The drawing under review shows one solid part. Ordinate dimensions are in mm from its lowest x, y, z. Give positions to 0.01 mm unless a question says otherwise; leave off trailing zeros. Order: outer loops, then holes, each group sorted by start corner. A loop starts at its lowest first (then second) coordinate and runs counter-clockwise, first axis right, second up. Notation, with made-up numbers: (64, -22.75) - (88, -22.75) arc R38 cw to (88, 15.25) - close; hole circle Ø10 at (-31, 58). An arc over 180 degrees is marked (long way). Write item = value, one per line. Start each with the question number.
1. We need section C-C, the plane z = 8.75. Give the boundary of the cut face in (x, y), and give its area (3 significant figures).
2. For P1, Ø0.9, axis at x = 2.5, y = 3, coming from the +Z side; P2, Ø2, axis at y = 1, z = 12, coming from the -X side; P3, Ø0.8, axis at y = 2, z = 0.5, coming from the -X side, all flat-tipped, find the tip position at first contact; note any pin that passes through.
3. Mouldability with a two-part tool opening along Y and no side actions: class the marked faces 1, 2 and 3 as pulls with the +Y half, pulls with the -Y half, needs draft (parallel to the pull), parting line crosses it, or undercut.
4. Wall thickness on probe 1 along Y at (x, z) = (3, 10); probe 2 along Z at (x, y) = (2.9, 1.65); probe 3 along Y at (x, z) = (4.1, 10.5): over which ranges is each line inside the solid? List them lowest first.
5. We need section D-D, the plane z = 4.25. Give the boundary of the cut face in (x, y).
6. We need section B-B, the plane x = 3. Give the boundary of the cut face in (y, z), and give its area (4 significant figures).
7. We need section A-A, the plane y = 3. Give the boundary of the cut face in (x, z).
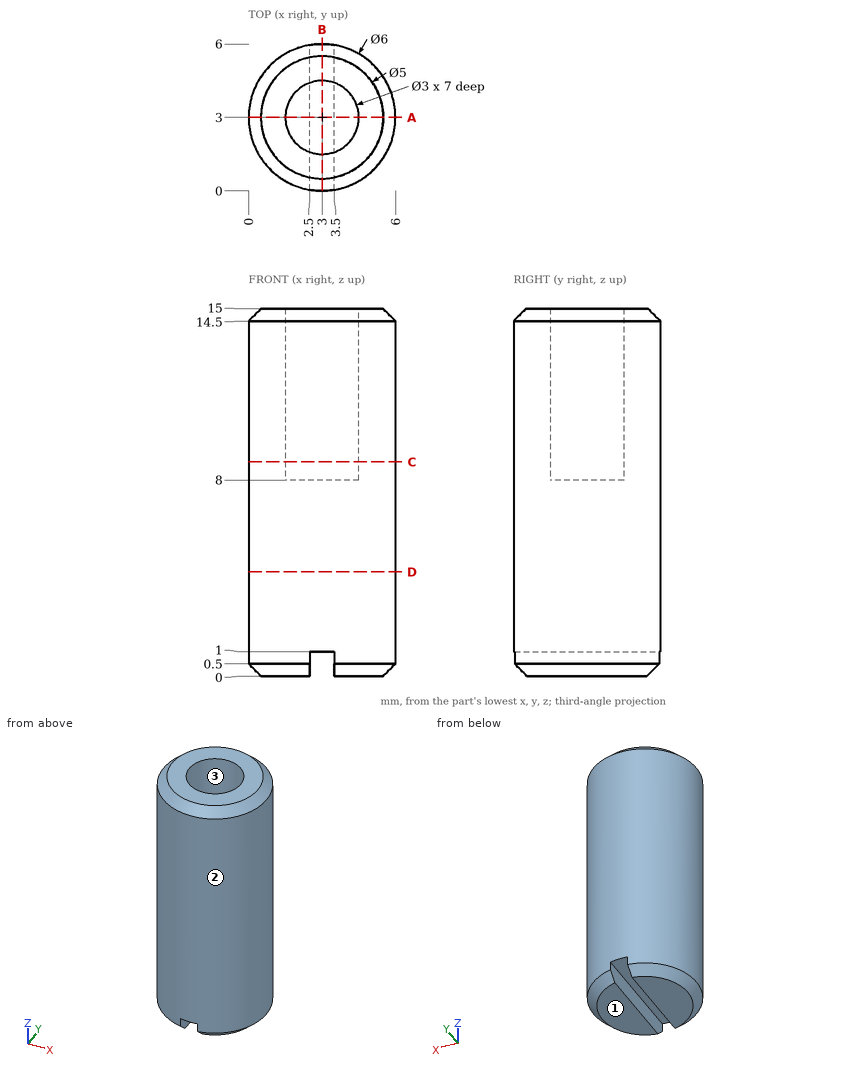
Model answer:
q1.outline = circle Ø6 at (3, 3); hole circle Ø3 at (3, 3)
q1.area = 21.2 mm2
q2.P1 = 8
q2.P2 = 0.17
q2.P3 = 0.06
q3.face_1 = needs draft
q3.face_2 = parting line crosses it
q3.face_3 = undercut
q4.probe_1 = 0 to 1.5, 4.5 to 6
q4.probe_2 = 1 to 8
q4.probe_3 = 0.21 to 1.98, 4.02 to 5.79
q5.outline = circle Ø6 at (3, 3)
q6.outline = (0, 1) - (6, 1) - (6, 14.5) - (5.5, 15) - (4.5, 15) - (4.5, 8) - (1.5, 8) - (1.5, 15) - (0.5, 15) - (0, 14.5) - close
q6.area = 62.75 mm2
q7.outline = (0, 0.5) - (0.5, 0) - (2.5, 0) - (2.5, 1) - (3.5, 1) - (3.5, 0) - (5.5, 0) - (6, 0.5) - (6, 14.5) - (5.5, 15) - (4.5, 15) - (4.5, 8) - (1.5, 8) - (1.5, 15) - (0.5, 15) - (0, 14.5) - close
